Check sheet for the modelled part. Datum: model origin and axes. Units: mm. Round coordinates to 2 decimals unless told otherwise and drop trailing zeros. Order: outer loops, then holes, each group sorted by start corner. A loop starts at its lowest first (then second) coordinate and runs counter-clockwise, first axis right, second up.
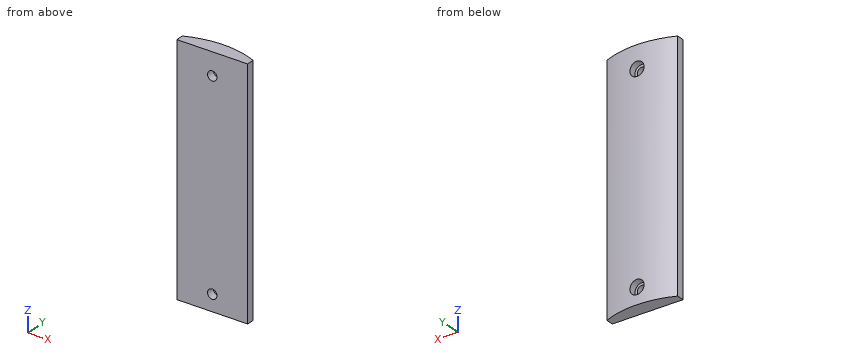
Autodesk Inventor part; units mm, degrees
ref_plane "YZ Plane" through (0, 0, 0) normal (1, 0, 0) x (0, 1, 0)
ref_plane "XZ Plane" through (0, 0, 0) normal (0, 1, 0) x (-1, 0, 0)
ref_plane "XY Plane" through (0, 0, 0) normal (0, 0, 1) x (1, 0, 0)
sketch "Sketch1" plane through (0, 0, 0) normal (0, 0, 1) x (1, 0, 0)
  line L0 (0, 0) -> (38.1, 0)
  arc A0 (33.6372, 3.2217) -> (3.5441, 3.2217) centre (18.5906, -30.8441) ccw
  line L1 (-11.7643, 6.3967) -> (19.5622, 6.3967) construction
  line L2 (-11.7643, 6.3967) -> (-11.7643, 0.0467) construction
  line L3 (3.5441, 3.2217) -> (3.5441, 0)
  line L4 (33.6372, 3.2217) -> (33.6372, 0)
  line L5 (3.5441, 0) -> (33.6372, 0)
  dimension "d0" = 38.1
  dimension "d1" = 6.35
extrude "Extrusion1" add sketch "Sketch1" along normal blind 101.6
ref_plane "Work Plane1" through (18.5906, 6.3967, 0) normal (0, -1, 0) x (1, 0, 0)
sketch "Sketch5" plane through (18.5906, 6.3967, 0) normal (0, -1, 0) x (1, 0, 0)
  point P0 (-18.5906, 0)
  point P1 (0, 6.9039)
  point P2 (0, 92.1664)
hole "Hole2" at (18.5906, 6.3967, 6.9039) at (18.5906, 6.3967, 92.1664) direction (0, -1, 0) diameter 4 end through all counterbore diameter 6 counterbore depth 3
properties part number "Beacon Push Bar"
Item 1: Scan lines: line 1 along Z through (x, y) = (18.5, 0.75); line 2 along Z through (x, y) = (19.5, 1); line 3 along Y through (x, z) = (19, 32). Record each from-to range of solid material in increasing order.
Answer:
line 1: z = 0 to 4.91, 8.9 to 90.17, 94.16 to 101.6
line 2: z = 0 to 5.12, 8.69 to 90.39, 93.95 to 101.6
line 3: y = 0 to 6.39
Item 2: Sectioned sample at B-B (y = 4.75). Record the cut outline in (x, z), and give its area (3 significant figures).
Answer:
outline: (7.64, 0) - (29.54, 0) - (29.54, 101.6) - (7.64, 101.6) - close; hole circle Ø6 at (18.59, 6.9); hole circle Ø6 at (18.59, 92.17)
area: 2,170 mm2
Item 3: Sectioned sample at A-A (z = 8). Record the cut outline in (x, y).
Answer:
outline: (3.54, 0) - (16.92, 0) - (16.92, 3.4) - (15.8, 3.4) - (15.8, 6.29) arc R37.24 ccw to (3.54, 3.22) - close; (20.26, 0) - (33.64, 0) - (33.64, 3.22) arc R37.24 ccw to (21.38, 6.29) - (21.38, 3.4) - (20.26, 3.4) - close
Item 4: Go/stop test with flat-tipped pins: P1, Ø5, axis at x = 18.59, z = 92.17, coming from the +Y side; P2, Ø1, axis at x = 7.5, z = 56, coming from the +Y side. Record where each tip stops, or that it passes through.
Answer:
P1: stops at y = 3.4
P2: stops at y = 4.86
Item 5: Sectioned sample at D-D (z = 40.5). Record the cut outline in (x, y), and give its area (3 significant figures).
Answer:
outline: (3.54, 0) - (33.64, 0) - (33.64, 3.22) arc R37.24 ccw to (3.54, 3.22) - close
area: 161 mm2
Item 6: Sectioned sample at C-C (x = 27.5). Record the cut outline in (y, z).
Answer:
outline: (0, 0) - (5.32, 0) - (5.32, 101.6) - (0, 101.6) - close
